Autodesk Inventor part; units mm, degrees
ref_plane "YZ Plane" through (0, 0, 0) normal (1, 0, 0) x (0, 1, 0)
ref_plane "XZ Plane" through (0, 0, 0) normal (0, 1, 0) x (-1, 0, 0)
ref_plane "XY Plane" through (0, 0, 0) normal (0, 0, 1) x (1, 0, 0)
sketch "Sketch1" plane through (0, 0, 0) normal (0, 1, 0) x (-1, 0, 0)
  line L0 (0, 0) -> (-10, 0)
  line L1 (-10, 0) -> (-10, -60)
  line L2 (-10, -60) -> (0, -60)
  line L3 (0, -60) -> (0, 0)
  dimension "d0" = 10
  dimension "d1" = 60
extrude "Extrusion1" add sketch "Sketch1" along normal blind 2.5
chamfer "Chamfer1" distance 0.002 angle 45 4 edges at (10, 0, -30) (5, 0, -60) (0, 0, -30) (5, 0, 0)
extrude "Extrusion2" add sketch "Sketch1" against normal blind 2.5
equation "\"d0\" = driveMagnet_width"
equation "\"d1\" = driveMagnet_length"
equation "\"d2\" = 0.5 * driveMagnet_height"
equation "\"d4\" = 0.5 * driveMagnet_height"
equation "\"gap\" = 0.1"
equation "\"airgap\" = 0.4"
equation "\"driveMagnet_length\" = 60"
equation "\"driveMagnet_width\" = 10"
equation "\"driveMagnet_height\" = 5"
equation "\"halbachMagnet_height\" = 3"
equation "\"sensorMagnet_diameter\" = 5"
equation "\"sensorMagnet_height\" = 2.66667"
equation "\"wallgap\" = 2"
equation "\"motorRadius\" = 2 * gap + driveMagnet_centerSpacingRadius + driveMagnet_length + 2 * wallgap"
equation "\"shaftDiameter\" = 8"
equation "\"flangeBearing_outerDiameter\" = 16"
equation "\"flangeBearing_innerDiameter\" = shaftDiameter"
equation "\"flangeBearing_height\" = 5"
equation "\"flangeBearing_flangeHeight\" = 1"
equation "\"flangeBearing_flangeDiameter\" = 18"
equation "\"magnetTrapNut_height\" = 1.2"
equation "\"magnetTrapNut_sideToSide\" = 4"
equation "\"magnetTrapBolt_headHeight\" = 2"
equation "\"magnetTrapBolt_headDiameter\" = 3.98"
equation "\"magnetTrapBolt_diameter\" = 2"
equation "\"statorThickness\" = coilThickness + 2 * wallgap"
equation "\"rotor_mountingLipHeight\" = 0.5 * statorThickness"
equation "\"magnetTrapHexNut_sideToSide\" = 4"
equation "\"magnetTrapSquareNut_sideLength\" = 4"
equation "\"magnetTrapSquareNut_height\" = 1.2"
equation "\"magnetTrapHexNut_height\" = 1.2"
equation "\"rotorRadius\" = 2 * gap + driveMagnet_centerSpacingRadius + driveMagnet_length + wallgap"
equation "\"rotorBandSquareNut_sideLength\" = 4"
equation "\"rotorBandHexNut_height\" = 1.2"
equation "\"rotorBandHexNut_sideToSide\" = 4"
equation "\"rotorBandSquareNut_height\" = 1.2"
equation "\"rotorBandBolt_headHeight\" = 2"
equation "\"rotorBandBolt_headDiameter\" = 3.98"
equation "\"rotorBandBolt_diameter\" = 2"
equation "\"rotorBandThickness\" = wallgap + rotorBandBolt_headHeight + gap"
equation "\"flangeCoupling_collarOuterDiameter\" = 16"
equation "\"flangeCoupling_flangeHoleEdgeToEdge\" = 2.05"
equation "\"flangeCoupling_innerDiameter\" = shaftDiameter"
equation "\"flangeCoupling_flangeHoleDiameter\" = 3.9"
equation "\"flangeCoupling_flangeHeight\" = 3.1"
equation "\"flangeCoupling_flangeDiameter\" = 32"
equation "\"flangeCoupling_height\" = flangeCoupling_collarHeight + flangeCoupling_flangeHeight"
equation "\"flangeCoupling_mountHoleDiameter\" = 3.9"
equation "\"flangeCoupling_mountHoleEdgeToEdge\" = 2.05"
equation "\"statorRadius\" = driveMagnet_length + driveMagnet_centerSpacingRadius + 2 * gap"
equation "\"coilThickness\" = 12"
equation "\"statorMountBolt_diameter\" = 4"
equation "\"statorMountBolt_headDiameter\" = 7"
equation "\"statorMountBolt_headHeight\" = 4"
equation "\"statorMountBolt_shaftLength\" = coilThickness + flangeCoupling_flangeHeight + wallgap"
equation "\"statorMountHexNut_height\" = 4"
equation "\"statorMountHexNut_sideToSide\" = 8"
equation "\"sensorMagnet_ringRadius\" = 0.5 * driveMagnet_centerSpacingRadius + 2 * wallgap"
equation "\"coil_percentCoverage\" = 0.6"
equation "\"statorSpokeDegrees\" = 4deg"
equation "\"coil_bulge\" = 3"
equation "\"statorCoilBolt_shaftLength\" = coilThickness"
equation "\"statorCoilHexNut_height\" = 1.2"
equation "\"statorCoilBolt_headHeight\" = 2"
equation "\"statorCoilBolt_diameter\" = 2"
equation "\"statorCoilBolt_headDiameter\" = 3.98"
equation "\"statorCoilHexNut_sideToSide\" = 4"
properties part number "DriveMagnet"
The model under review builds one solid part; all positions refer to its coordinate system, in mm. Round coordinates to 2 decimals unless told otherwise and drop trailing zeros. Write each question's results on one line, items separated by ' | '. Start each with the question number.
Q1. Insertion check: P1, Ø1, axis at y = -2, z = -8, coming from the -X side. The pin has a flat end and moves straight along its axis. Give the tip position at first contact, or say it passes through.
Q2. Wall thickness on line 1 along X through (y, z) = (0, -43): over which ranges is the line inside the solid? List them lowest first. Write a range as [from, to].
Q3. Draft analysis for pull direction Y (two halves, no side actions). For faces 1 (the flat face through (5, 2.5, -30)), 2 (the flat face through (5, -1, 0)), 3 (the flat face through (5, -2.5, -30)), state which applies: pulls with the +Y half, pulls with the -Y half, needs draft (parallel to the pull), parting line crosses it, or undercut.
Data:
1) P1: stops at x = 0
2) line 1: x = [0, 10]
3) face 1: pulls with the +Y half | face 2: needs draft | face 3: pulls with the -Y half
